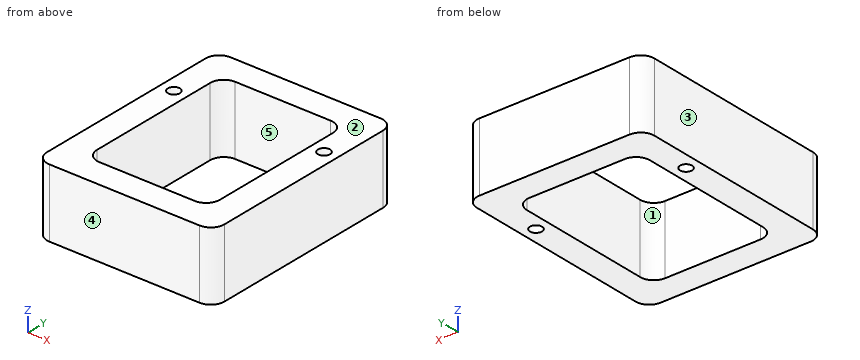
```python
from build123d import *

# Parameters (mm, degrees)
SKETCH1_R           = 11.2
BOSS_EXTRUDE1_DEPTH = 127


with BuildPart() as part:
    # Sketch1 → Boss-Extrude1 (new body)
    with BuildSketch(Plane.XY):
        with BuildLine():
            Line((-139.7, -203.2), (139.7, -203.2))
            ThreePointArc((139.7, -203.2), (157.660512242, -195.760512242), (165.1, -177.8))
            Line((165.1, -177.8), (165.1, 177.8))
            ThreePointArc((165.1, 177.8), (157.660512242, 195.760512242), (139.7, 203.2))
            Line((139.7, 203.2), (-139.7, 203.2))
            ThreePointArc((-139.7, 203.2), (-157.660512242, 195.760512242), (-165.1, 177.8))
            Line((-165.1, 177.8), (-165.1, -177.8))
            ThreePointArc((-165.1, -177.8), (-157.660512242, -195.760512242), (-139.7, -203.2))
        make_face()
        with Locations((-139.7, 76.2)):
            Circle(SKETCH1_R, mode=Mode.SUBTRACT)
        with Locations((139.7, 76.2)):
            Circle(SKETCH1_R, mode=Mode.SUBTRACT)
        with BuildLine():
            Line((-114.3, -127), (-114.3, 127))
            ThreePointArc((-114.3, 127), (-106.860512242, 144.960512242), (-88.9, 152.4))
            Line((-88.9, 152.4), (88.9, 152.4))
            ThreePointArc((88.9, 152.4), (106.860512242, 144.960512242), (114.3, 127))
            Line((114.3, 127), (114.3, -127))
            ThreePointArc((114.3, -127), (106.860512242, -144.960512242), (88.9, -152.4))
            Line((88.9, -152.4), (-88.9, -152.4))
            ThreePointArc((-88.9, -152.4), (-106.860512242, -144.960512242), (-114.3, -127))
        make_face(mode=Mode.SUBTRACT)
    extrude(amount=BOSS_EXTRUDE1_DEPTH)


solid = part.part
```
Design review of the part built by this model. Coordinates are the model's own, in mm. Face numbers are marked on the shaded views. A direction names the side the tool comes from. Give positions to 0.01 mm unless a question says otherwise; leave off trailing zeros. Write each loop counter-clockwise with the first axis right and the second up, starting at its lowest first coordinate (ties: lowest second). Pieces come first, ordered by that corner, then holes. Notation, with made-up numbers: (53.5, 19) - (98.5, 19) arc R19 ccw to (98.5, 25) - close; hole circle Ø2 at (-31, 52). An arc over 180 degrees is marked (long way). Return JSON: item names as keys, results as strings. Group by question number.
(1) We need section C-C, the plane y = -108. Give the boundary of the cut face in (x, z), then the cut area to 3 significant figures.
(2) We need section B-B, the plane x = -51. Give the boundary of the cut face in (y, z), then the cut area to 3 significant figures.
(3) Insertion check: pin 1 (13.5 mm diameter, centred on x = 139.7, y = 76.2, fed in from -Z). The pin has a flat end and moves straight along its axis. Give the tip position at first contact, or say it passes through.
(4) We need section D-D, the plane z = 39. Give the boundary of the cut face in (x, y).
(5) We need section A-A, the plane y = 76.2. Give the boundary of the cut face in (x, z), then the cut area to 3 significant figures.
(6) Machinability: for the marked faces 1 and 2, which of the approach directions +Z, -Z, +X, -X, +Y, -Y give a long, thin tool a straight path to every point of the face, cutting with its end or side? Answer none if there is none.
(7) Mouldability with a two-part tool opening along Y and no side actions: class the marked faces 3, 4 and 5 as +Y half, -Y half, draft (parallel to the pull), parting line (faces both ways), or undercut.
(8) To check wall thickness, follow probe 1 along X at (y, z) = (76, 95); probe 2 along Y at (x, z) = (38.5, 103); probe 3 along X at (y, z) = (42.5, 91). State the ranges of each line that lie inside material, in increasing order.
Reported:
{
 "1": {"outline": "(-165.1, 0) - (-114.3, 0) - (-114.3, 127) - (-165.1, 127) - close; (114.3, 0) - (165.1, 0) - (165.1, 127) - (114.3, 127) - close", "area": "12,900 mm2"},
 "2": {"outline": "(-203.2, 0) - (-152.4, 0) - (-152.4, 127) - (-203.2, 127) - close; (152.4, 0) - (203.2, 0) - (203.2, 127) - (152.4, 127) - close", "area": "12,900 mm2"},
 "3": {"pin 1": "passes through"},
 "4": {"outline": "(-165.1, -177.8) arc R25.4 ccw to (-139.7, -203.2) - (139.7, -203.2) arc R25.4 ccw to (165.1, -177.8) - (165.1, 177.8) arc R25.4 ccw to (139.7, 203.2) - (-139.7, 203.2) arc R25.4 ccw to (-165.1, 177.8) - close; hole circle Ø22.4 at (-139.7, 76.2); hole (-114.3, -127) arc R25.4 ccw to (-88.9, -152.4) - (88.9, -152.4) arc R25.4 ccw to (114.3, -127) - (114.3, 127) arc R25.4 ccw to (88.9, 152.4) - (-88.9, 152.4) arc R25.4 ccw to (-114.3, 127) - close; hole circle Ø22.4 at (139.7, 76.2)"},
 "5": {"outline": "(-165.1, 0) - (-150.9, 0) - (-150.9, 127) - (-165.1, 127) - close; (-128.5, 0) - (-114.3, 0) - (-114.3, 127) - (-128.5, 127) - close; (114.3, 0) - (128.5, 0) - (128.5, 127) - (114.3, 127) - close; (150.9, 0) - (165.1, 0) - (165.1, 127) - (150.9, 127) - close", "area": "7,210 mm2"},
 "6": {"face 1": "+Z, -Z", "face 2": "+Z, +X, -X, +Y, -Y"},
 "7": {"face 3": "draft", "face 4": "-Y half", "face 5": "undercut"},
 "8": {"probe 1": "x = -165.1 to -150.9, -128.5 to -114.3, 114.3 to 128.5, 150.9 to 165.1", "probe 2": "y = -203.2 to -152.4, 152.4 to 203.2", "probe 3": "x = -165.1 to -114.3, 114.3 to 165.1"}
}
